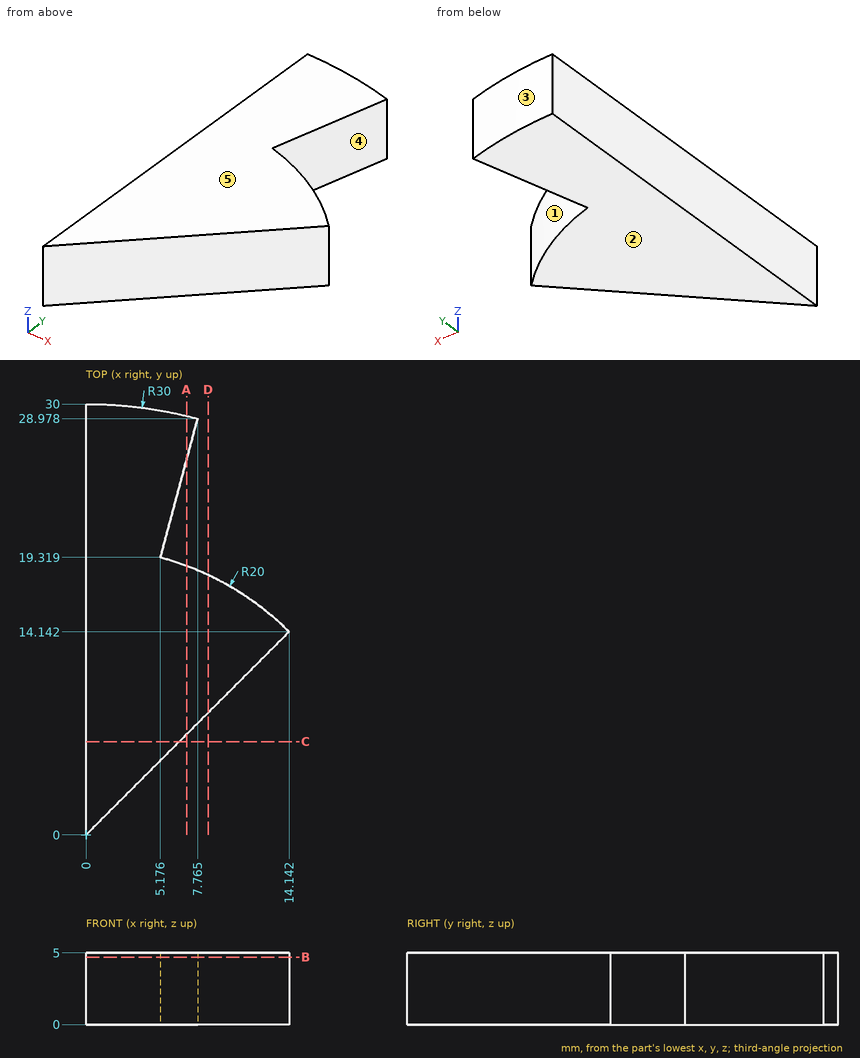
Here's the drawing with two shaded views (mm, measured from the low corner). I have some questions. A direction names the side the tool comes from. Give positions to 0.01 mm unless a question says otherwise; leave off trailing zeros. Order: outer loops, then holes, each group sorted by start corner. A loop starts at its lowest first (then second) coordinate and runs counter-clockwise, first axis right, second up. Notation, with made-up numbers: M -16.5,22 L 11.5,22 A27 cw 11.5,38 Z; hole C -1.75,-21.5 d5. An arc over 180 degrees is marked long. One line per item, written item: value.
1) For P1, Ø2, axis at x = 2.5, z = 2, coming from the +Y side, with a flat end and sliding along its axis, tell me the tip position at first contact or that it passes through.
Answer sheet:
P1: stops at y = 29.96
2) I want a section at A-A, the plane x = 7. List the corners of the cut face in (y, z) for me (1 decimal).
Answer sheet:
outline: M 7,0 L 18.7,0 L 18.7,5 L 7,5 Z; M 26.1,0 L 29.2,0 L 29.2,5 L 26.1,5 Z
3) We'd pull the mould along Y, two halves only. Please class the marked faces 3, 4 and 5: released by +Y, released by -Y, zero draft, split by the parting line, or undercut.
Answer sheet:
face 3: released by +Y
face 4: undercut
face 5: zero draft
4) I want a section at D-D, the plane x = 8.5. List the corners of the cut face in (y, z) for me.
Answer sheet:
outline: M 8.5,0 L 18.1,0 L 18.1,5 L 8.5,5 Z
5) I want a section at C-C, the plane y = 6.5. List the corners of the cut face in (x, z) for me.
Answer sheet:
outline: M 0,0 L 6.5,0 L 6.5,5 L 0,5 Z
6) I want a section at B-B, the plane z = 4.7. List the corners of the cut face in (x, y) for me (1 decimal).
Answer sheet:
outline: M 0,0 L 14.1,14.1 A20 ccw 5.2,19.3 L 7.8,29 A30 ccw 0,30 Z
7) Please list where these lines run through material, in increasing order: line 1 along X through (y, z) = (7.5, 4.6); line 2 along X through (y, z) = (6.25, 0.4); line 3 along Y through (x, z) = (1.75, 3.6).
Answer sheet:
line 1: x = 0 to 7.5
line 2: x = 0 to 6.25
line 3: y = 1.75 to 29.95
8) On a 3-axis mill with a long thin cutter (end or side, diameter ignored), from which of +Z, -Z, +X, -X, +Y, -Y can I reach the whole of each face in a straight line? I mean the marked faces 1 and 2. Say none if no direction works.
Answer sheet:
face 1: +Z, -Z, +X
face 2: -Z, +X, -X, +Y, -Y
